Autodesk Fusion 360 part; units mm, degrees
sketch "Sketch1" plane through (0, 0, 0) normal (1, 0, 0) x (0, 1, 0)
  circle A0 centre (0, 0) radius 17.5
  line L0 (0, 0) -> (0, 17.5)
  dimension "d1" = 35
extrude "Extrude1" add sketch "Sketch1" along normal blind 40
sketch "Sketch2" plane through (40, 0, 0) normal (1, 0, 0) x (0, 1, 0)
  circle A0 centre (0, 0) radius 17.5
  circle A1 centre (0, 0) radius 18.5
  point P0 (0, 7)
  dimension "d5" = 37
extrude "Extrude2" add sketch "Sketch2" along normal blind 20 contours A0 | A1
sketch "Sketch3" plane through (60, 0, 0) normal (1, 0, 0) x (0, 1, 0)
  circle A0 centre (0, 0) radius 18.5
  line L0 (0, 0) -> (0, 7)
  circle A1 centre (0, 7) radius 6
  circle A2 centre (0, 0) radius 15.5 construction
  line L1 (0, 0) -> (0, 15.5)
  circle A3 centre (-15.4999, -0.0425) radius 1.5
  circle A4 centre (-7.7132, -13.4446) radius 1.5
  circle A5 centre (7.7868, -13.4021) radius 1.5
  circle A6 centre (15.4999, 0.0425) radius 1.5
  circle A7 centre (7.7132, 13.4446) radius 1.5
  circle A8 centre (-7.7868, 13.4021) radius 1.5
  dimension "d8" = 12
  dimension "d9" = 31
  dimension "d10" = 3
  dimension "d12" = 360
extrude "Extrude3" cut sketch "Sketch3" against normal blind 3 contours A3 | A4 | A5 | A6 | A7 | A8
sketch "Sketch4" plane through (60, 0, 0) normal (1, 0, 0) x (0, 1, 0)
  circle A0 centre (7.7868, -13.4021) radius 1.5
  circle A1 centre (-7.7868, 13.4021) radius 1.5
  circle A2 centre (15.4999, 0.0425) radius 1.5
  circle A3 centre (-7.7132, -13.4446) radius 1.5
  circle A4 centre (-15.4999, -0.0425) radius 1.5
  circle A5 centre (7.7132, 13.4446) radius 1.5
  circle A6 centre (0, 0) radius 18.5
  circle A7 centre (0, 0) radius 18.5
  line L0 (0, 0) -> (0, 7) construction
  circle A8 centre (0, 7) radius 6
  dimension "d15" = 37
  dimension "d16" = 7
  dimension "d17" = 12
extrude "Extrude4" add sketch "Sketch4" along normal blind 6 contours A8
sketch "Sketch6" plane through (66, 0, 0) normal (1, 0, 0) x (0, 1, 0)
  circle A0 centre (0, 7) radius 6
  circle A1 centre (0, 7) radius 3
  dimension "d21" = 6
extrude "Extrude5" add sketch "Sketch6" along normal blind 12.3 contours A1
Geometry check sheet. Reference: the model listing, model coordinates, mm. A direction names the side the tool comes from. Round coordinates to 2 decimals unless told otherwise and drop trailing zeros. Loops run counter-clockwise (first coordinate to the right, second up) from the corner with the lowest first, then second, coordinate; pieces in that order, holes last. Notation, with made-up numbers: (42.5, -5) - (61.5, -5) arc R18 cw to (61.5, 6) - close; hole circle Ø6 at (83, 81.5). An arc over 180 degrees is marked (long way). Answer as CSV lines item,"result".
(1) Cross-section at D-D, the plane x = 15.5. Enter the section's corners in (y, z), and give its area (3 significant figures).
Output values:
outline,"circle Ø35 at (0, 0)"
area,"962 mm²"
(2) Set-up check for faces 4 (the face through (40, -11, -14)), 5 (the face through (58.521, 9.144, 13.895)), 6 (the face through (0, 0, 0)): record each of +Z, -Z, +X, -X, +Y, -Y from which the full face is reachable in a straight line by a thin tool's end or side.
Output values:
face 4,"-X"
face 5,"+X"
face 6,"+Z, -Z, -X, +Y, -Y"
(3) Cross-section at C-C, the plane z = -6.5. Enter the section's corners in (x, y), and give its area (3 significant figures).
Output values:
outline,"(0, -16.25) - (40, -16.25) - (40, -17.32) - (60, -17.32) - (60, 17.32) - (40, 17.32) - (40, 16.25) - (0, 16.25) - close"
area,"1,990 mm²"
(4) Depth check by flat-ended pin: pin 1 Ø1.5 at (x, z) = (43, -3) entering from -Y; pin 2 Ø1.5 at (y, z) = (-8.5, 13) entering from +X; pin 3 Ø0.9 at (y, z) = (8, -13.5) entering from +X. Enter the tip coordinate at first touch or a pass-through.
Output values:
pin 1,"stops at y = -18.36"
pin 2,"stops at x = 60"
pin 3,"stops at x = 57"
(5) Cross-section at B-B, the plane y = 0. Enter the section's corners in (x, z), and give its area (3 significant figures).
Output values:
outline,"(0, -17.5) - (40, -17.5) - (40, -18.5) - (60, -18.5) - (60, 1) - (66, 1) - (66, 4) - (78.3, 4) - (78.3, 10) - (66, 10) - (66, 13) - (60, 13) - (60, 18.5) - (40, 18.5) - (40, 17.5) - (0, 17.5) - close"
area,"2,290 mm²"
(6) Cross-section at A-A, the plane x = 58. Enter the section's corners in (y, z), and give its area (3 significant figures).
Output values:
outline,"circle Ø37 at (0, 0); hole circle Ø3 at (-15.5, -0.04); hole circle Ø3 at (-7.79, 13.4); hole circle Ø3 at (-7.71, -13.44); hole circle Ø3 at (7.71, 13.44); hole circle Ø3 at (7.79, -13.4); hole circle Ø3 at (15.5, 0.04)"
area,"1,030 mm²"
(7) Release check for a two-part mould opening along Y. For faces 1 (the face through (19.72, -13.887, 10.648)), 2 (the face through (78.3, 0, 7)), 3 (the face through (58.521, -6.356, 13.853)) record: released by +Y, released by -Y, zero draft, split by the parting line, or undercut.
Output values:
face 1,"split by the parting line"
face 2,"zero draft"
face 3,"undercut"
(8) Material ranges on line 1 along X through (y, z) = (-7.5, -3); line 2 along X through (y, z) = (-7, 14); line 3 along Z through (x, y) = (57, 0), recorded low to high.
Output values:
line 1,"x = 0 to 60"
line 2,"x = 0 to 57"
line 3,"z = -18.5 to 18.5"
